from build123d import *

# Parameters (mm, degrees)
BOSS_EXTRUDE1_DEPTH = 28


with BuildPart() as part:
    # Sketch1 → Boss-Extrude1 (new body)
    with BuildSketch(Plane.XY):
        with BuildLine():
            Line((-3, -5), (3, -5))
            Line((3, -5), (3, -6.5))
            ThreePointArc((3, -6.5), (4.5, -8), (6, -6.5))
            Line((6, -6.5), (6, -5))
            Line((6, -5), (6, 5))
            Line((6, 5), (-6, 5))
            Line((-6, 5), (-6, -5))
            Line((-6, -5), (-6, -6.5))
            ThreePointArc((-6, -6.5), (-4.5, -8), (-3, -6.5))
            Line((-3, -6.5), (-3, -5))
        make_face()
    extrude(amount=BOSS_EXTRUDE1_DEPTH)


solid = part.part
Here's how the part is built. I have some questions about the finished solid (model axes, mm). A direction names the side the tool comes from. Round coordinates to 2 decimals unless told otherwise and drop trailing zeros. Write each loop counter-clockwise with the first axis right and the second up, starting at its lowest first coordinate (ties: lowest second). Pieces come first, ordered by that corner, then holes. Notation, with made-up numbers: (-12.5, -15.75) -> (-5.5, -15.75) arc R15 cw to (-5.5, -9.75) -> close; hole circle Ø3 at (8.25, -15.75). An arc over 180 degrees is marked (long way). One line per item, written item: value.
1) We'd pull the mould along X, two halves only. Please class faces 1 (the face through (6, -1, 14)), 2 (the face through (-6, -1, 14)), 3 (the face through (0, -1, 0)), 4 (the face through (0, -5, 14)): released by +X, released by -X, zero draft, split by the parting line, or undercut.
Filled sheet:
face 1: released by +X
face 2: released by -X
face 3: zero draft
face 4: undercut
2) I'm going to push flat-ended pins straight in: pin 1 Ø5 at (x, z) = (1, 8) entering from -Y; pin 2 Ø1.5 at (x, z) = (2, 11.5) entering from -Y. Where does each tip first touch, or does it pass through?
Filled sheet:
pin 1: stops at y = -7.62
pin 2: stops at y = -5
3) If I drill on line 1 (X direction, y = -6.5, z = 10.5); line 2 (Y direction, x = -2, z = 15.75); line 3 (Y direction, x = 4, z = 17), over which ranges is the centre line in solid material (lowest first)? Write a range as [from, to].
Filled sheet:
line 1: x = [-6, -3], [3, 6]
line 2: y = [-5, 5]
line 3: y = [-7.91, 5]
4) Suppose I cut it at A-A on z = 4. List the corners of the cut face in (x, y) for me, plus the area to 3 significant figures.
Filled sheet:
outline: (-6, -6.5) arc R1.5 ccw to (-3, -6.5) -> (-3, -5) -> (3, -5) -> (3, -6.5) arc R1.5 ccw to (6, -6.5) -> (6, 5) -> (-6, 5) -> close
area: 136 mm2
5) Suppose I cut it at B-B on x = 3.5. List the corners of the cut face in (y, z) for me, plus the area to 3 significant figures.
Filled sheet:
outline: (-7.62, 0) -> (5, 0) -> (5, 28) -> (-7.62, 28) -> close
area: 353 mm2
6) For faces 5 (the face through (0, 5, 14)), 6 (the face through (-3, -6, 14)), which set-ups out of +Z, -Z, +X, -X, +Y, -Y let a thin tool reach every point of the face, with its end or its side?
Filled sheet:
face 5: +Z, -Z, +X, -X, +Y
face 6: +Z, -Z, -Y
